from build123d import *

# Parameters (mm, degrees)
SKETCH_1_W      = 412.9
SKETCH_1_H      = 81.4
SKETCH_1_R      = 2
EXTRUDE_1_DEPTH = 0.6
SKETCH_2_R      = 2
EXTRUDE_2_DEPTH = 0.6
EXTRUDE_START   = -0.6
SKETCH_3_R      = 2
EXTRUDE_3_DEPTH = 0.6


with BuildPart() as part:
    # Эскиз1 → Бобышка-Вытянуть1 (new body)
    with BuildSketch(Plane.XY):
        with Locations((241.1, 40.7)):
            Rectangle(SKETCH_1_W, SKETCH_1_H)
        with Locations((40.25, 10.7)):
            Circle(SKETCH_1_R, mode=Mode.SUBTRACT)
        with Locations((441.95, 10.7)):
            Circle(SKETCH_1_R, mode=Mode.SUBTRACT)
        with Locations((40.25, 40.7)):
            Circle(SKETCH_1_R, mode=Mode.SUBTRACT)
        with Locations((40.25, 70.7)):
            Circle(SKETCH_1_R, mode=Mode.SUBTRACT)
        with Locations((441.95, 40.7)):
            Circle(SKETCH_1_R, mode=Mode.SUBTRACT)
        with Locations((441.95, 70.7)):
            Circle(SKETCH_1_R, mode=Mode.SUBTRACT)
    extrude(amount=EXTRUDE_1_DEPTH)

    # Эскиз2 → Бобышка-Вытянуть2 (add)
    with BuildSketch(Plane(origin=(0, 81.4, 0), x_dir=(1, 0, 0), z_dir=(0, 1, 0))):
        Polygon((44.65, -0.6), (50.423502692, -10.6), (431.776497308, -10.6), (437.55, -0.6), align=None)
        with Locations(Location((401.1, -5.6, 0), (0, 0, 180))):
            Circle(SKETCH_2_R, mode=Mode.SUBTRACT)
        with Locations(Location((321.1, -5.6, 0), (0, 0, 180))):
            Circle(SKETCH_2_R, mode=Mode.SUBTRACT)
        with Locations(Location((241.1, -5.6, 0), (0, 0, 180))):
            Circle(SKETCH_2_R, mode=Mode.SUBTRACT)
        with Locations(Location((161.1, -5.6, 0), (0, 0, 180))):
            Circle(SKETCH_2_R, mode=Mode.SUBTRACT)
        with Locations(Location((81.1, -5.6, 0), (0, 0, 180))):
            Circle(SKETCH_2_R, mode=Mode.SUBTRACT)
    extrude(amount=-EXTRUDE_2_DEPTH)

    # Эскиз3 → Бобышка-Вытянуть3 (add)
    with BuildSketch(Plane.XZ.offset(EXTRUDE_START)):
        Polygon((44.65, 0.6), (437.55, 0.6), (431.776497308, 10.6), (50.423502692, 10.6), align=None)
        with Locations(Location((401.1, 5.6, 0), (0, 0, 180))):
            Circle(SKETCH_3_R, mode=Mode.SUBTRACT)
        with Locations(Location((321.1, 5.6, 0), (0, 0, 180))):
            Circle(SKETCH_3_R, mode=Mode.SUBTRACT)
        with Locations(Location((241.1, 5.6, 0), (0, 0, 180))):
            Circle(SKETCH_3_R, mode=Mode.SUBTRACT)
        with Locations(Location((161.1, 5.6, 0), (0, 0, 180))):
            Circle(SKETCH_3_R, mode=Mode.SUBTRACT)
        with Locations(Location((81.1, 5.6, 0), (0, 0, 180))):
            Circle(SKETCH_3_R, mode=Mode.SUBTRACT)
    extrude(amount=EXTRUDE_3_DEPTH)


solid = part.part
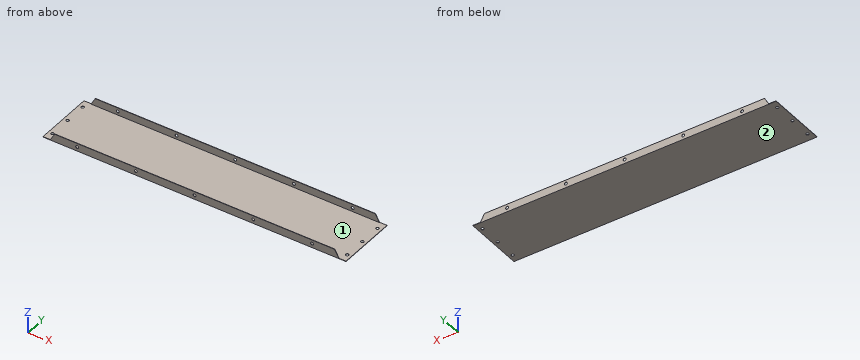
Geometry: final body of the model. Coordinates: model frame, mm. Face numbers are marked on the shaded views. Give positions to 0.01 mm unless a question says otherwise; leave off trailing zeros. Loops run counter-clockwise (first coordinate to the right, second up) from the corner with the lowest first, then second, coordinate; pieces in that order, holes last. Notation, with made-up numbers: (39, 30) - (64, 30) arc R11 cw to (64, 34) - close; hole circle Ø1 at (-7, 19). An arc over 180 degrees is marked (long way). Answer as CSV lines item,"result". Start each with the question number.
1. Draft query along Y for the marked faces 1 and 2. Return one class per face: released by +Y, released by -Y, zero draft, split by the parting line, or undercut.
2. Ray query, L1, parallel to Y at x = 40.25, z = 0.45; L2, parallel to Y at x = 124, z = 2.25; L3, parallel to Z at x = 247.5, y = 57.5. Return the intervals inside material, ascending.
3. Pin query (flat end, axial travel): P1, Ø6.5, axis at x = 40.25, y = 70.7, coming from the +Z side; P2, Ø6, axis at y = 21.5, z = 1.5, coming from the +X side. Return the tip coordinate at first contact, or that it passes through.
4. Section B-B, the plane y = 46.5. Return loops of the section in (x, z), plus the area to 3 significant figures.
5. Section A-A, the plane x = 393. Return loops of the section in (y, z).
Answers:
1,face 1,"undercut"
1,face 2,"zero draft"
2,L1,"y = 0 to 8.7, 12.7 to 38.7, 42.7 to 68.7, 72.7 to 81.4"
2,L2,"y = 0 to 0.6, 80.8 to 81.4"
2,L3,"z = 0 to 0.6"
3,P1,"stops at z = 0.6"
3,P2,"stops at x = 447.55"
4,outline,"(34.65, 0) - (447.55, 0) - (447.55, 0.6) - (34.65, 0.6) - close"
4,area,"248 mm2"
5,outline,"(0, 0) - (81.4, 0) - (81.4, 10.6) - (80.8, 10.6) - (80.8, 0.6) - (0.6, 0.6) - (0.6, 10.6) - (0, 10.6) - close"
